Part print with two shaded views. Sizes in mm from the minimum x, y, z corner. A direction names the side the tool comes from. Give positions to 0.01 mm unless a question says otherwise; leave off trailing zeros. Order: outer loops, then holes, each group sorted by start corner. A loop starts at its lowest first (then second) coordinate and runs counter-clockwise, first axis right, second up. Notation, with made-up numbers: M 12,1.25 L 66,1.25 A10 cw 66,20.25 Z; hole C -35.75,87 d10. An arc over 180 degrees is marked long. Return JSON: item names as keys, results as strings.
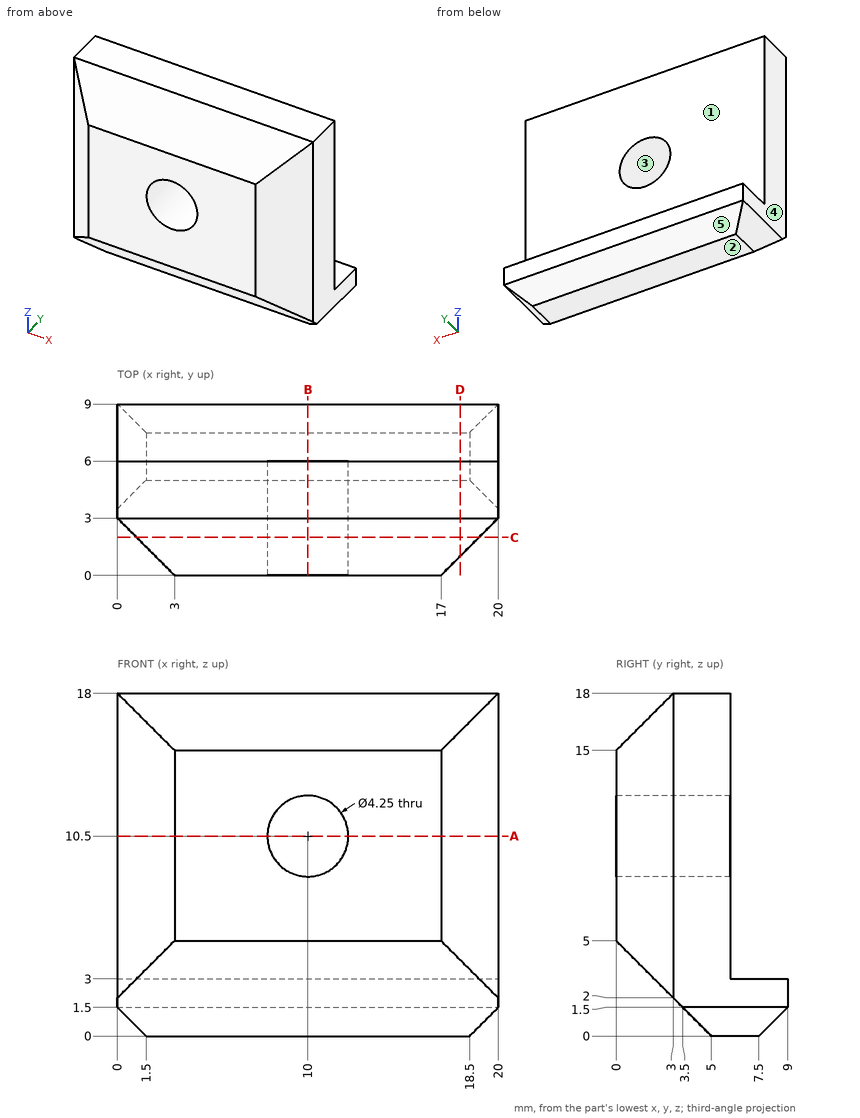
Q1. Probe line 1 along Y through (x, z) = (16.75, 9.5); line 2 along Z through (x, y) = (1.25, 2); line 3 along Z through (x, y) = (10, 4.3) (3 decimals). List the from-to ranges inside material, lowest first.
Established:
{"line 1": "y = 0 to 6", "line 2": "z = 3 to 17", "line 3": "z = 0.7 to 8.375, 12.625 to 18"}
Q2. Band-saw the part on D-D (x = 18). Give the cut face in (y, z), then the cut area to 3 significant figures.
Established:
{"outline": "M 1,4 L 5,0 L 7.5,0 L 9,1.5 L 9,3 L 6,3 L 6,18 L 3,18 L 1,16 Z", "area": "87.9 mm²"}
Q3. Band-saw the part on A-A (z = 10.5). Give the cut face in (x, y) (3 decimals), then the cut area to 3 significant figures.
Established:
{"outline": "M 0,3 L 3,0 L 7.875,0 L 7.875,6 L 0,6 Z; M 12.125,0 L 17,0 L 20,3 L 20,6 L 12.125,6 Z", "area": "85.5 mm²"}
Q4. Band-saw the part on C-C (y = 2). Give the cut face in (x, z) (3 decimals).
Established:
{"outline": "M 1,3 L 19,3 L 19,17 L 1,17 Z; hole C 10,10.5 d4.25"}
Q5. Band-saw the part on B-B (x = 10). Give the cut face in (y, z) (3 decimals), then the cut area to 3 significant figures.
Established:
{"outline": "M 0,5 L 5,0 L 7.5,0 L 9,1.5 L 9,3 L 6,3 L 6,8.375 L 0,8.375 Z; M 0,12.625 L 6,12.625 L 6,18 L 3,18 L 0,15 Z", "area": "73.4 mm²"}
Q6. Two-plate mould, pull along Z, no slides. Class the marked faces 3, 4 and 5: +Z half, -Z half, draft (parallel to the pull), parting line (faces both ways), or undercut.
Established:
{"face 3": "undercut", "face 4": "draft", "face 5": "-Z half"}
Q7. Pin check, flat tips, straight feed: pin 1 (5 mm diameter, centred on x = 10, z = 10.5, fed in from -Y); pin 2 (1 mm diameter, centred on y = 2, z = 14.5, fed in from -X); pin 3 (1 mm diameter, centred on x = 17.5, z = 9, fed in from +Y); pin 4 (2 mm diameter, centred on x = 11.5, z = 3.5, fed in from -Y). Stop position of each tip, or through.
Established:
{"pin 1": "stops at y = 0", "pin 2": "stops at x = 0.5", "pin 3": "stops at y = 6", "pin 4": "stops at y = 0.5"}
Q8. 3-axis set-ups, long thin cutter, end or side, ignore diameter. For the marked faces 1 and 2: which of +Z, -Z, +X, -X, +Y, -Y reach the whole face in a straight line?
Established:
{"face 1": "+Z, +X, -X, +Y", "face 2": "-Z, +X, -X, +Y, -Y"}
